from build123d import *

# Parameters (mm, degrees)
BOSS_EXTRUDE1_DEPTH     = 8
CUT_EXTRUDE1_DEPTH      = 2
CUT_EXTRUDE2_DEPTH      = 1
CUT_EXTRUDE2_DEPTH_BACK = 1
SKETCH7_R               = 0.5
BOSS_EXTRUDE4_DEPTH     = 30
CUT_EXTRUDE3_DEPTH      = 2


with BuildPart() as part:
    # Sketch1 → Boss-Extrude1 (new body)
    with BuildSketch(Plane(origin=(0, 0, 0), x_dir=(1, 0, 0), z_dir=(0, 1, 0))):
        with BuildLine():
            Line((12.297414328, 5.987472362), (16.301582158, 4.720916174))
            ThreePointArc((16.301582158, 4.720916174), (16.806716232, 4.358414998), (17, 3.767475981))
            Line((17, 3.767475981), (17, -3.767475981))
            ThreePointArc((17, -3.767475981), (16.806716232, -4.358414998), (16.301582158, -4.720916174))
            Line((16.301582158, -4.720916174), (12.297414328, -5.987472362))
            ThreePointArc((12.297414328, -5.987472362), (10.950566944, -6.649754843), (9.860946513, -7.68190952))
            ThreePointArc((9.860946513, -7.68190952), (-12.5, 0), (9.860946513, 7.68190952))
            ThreePointArc((9.860946513, 7.68190952), (10.950566944, 6.649754843), (12.297414328, 5.987472362))
        make_face()
    extrude(amount=BOSS_EXTRUDE1_DEPTH)

    # Sketch2 → Cut-Extrude1 (cut)
    with BuildSketch(Plane.XZ):
        with BuildLine():
            Line((1, 11.25), (1, 12.459935794))
            ThreePointArc((1, 12.459935794), (0, 12.5), (-1, 12.459935794))
            Line((-1, 12.459935794), (-1, 11.25))
            ThreePointArc((-1, 11.25), (0, 10.25), (1, 11.25))
        make_face()
        with BuildLine():
            Line((-11.25, -1), (-12.459935794, -1))
            ThreePointArc((-12.459935794, -1), (-12.5, 0), (-12.459935794, 1))
            Line((-12.459935794, 1), (-11.25, 1))
            ThreePointArc((-11.25, 1), (-10.25, 0), (-11.25, -1))
        make_face()
        with BuildLine():
            Line((1, -11.25), (1, -12.459935794))
            ThreePointArc((1, -12.459935794), (0, -12.5), (-1, -12.459935794))
            Line((-1, -12.459935794), (-1, -11.25))
            ThreePointArc((-1, -11.25), (0, -10.25), (1, -11.25))
        make_face()
    extrude(amount=-CUT_EXTRUDE1_DEPTH, mode=Mode.SUBTRACT)

    # Sketch3 → Cut-Extrude2 (cut, two sides: drawn at the far end of the back side and taken through both)
    with BuildSketch(Plane.XY.offset(-CUT_EXTRUDE2_DEPTH_BACK)):
        with BuildLine():
            Line((16, 0), (14.339588828, 3.617029189))
            ThreePointArc((14.339588828, 3.617029189), (14.248707164, 3.675309612), (14.1578255, 3.617029189))
            Line((14.1578255, 3.617029189), (12.497414328, 0))
            Line((12.497414328, 0), (16, 0))
        make_face()
    extrude(amount=CUT_EXTRUDE2_DEPTH + CUT_EXTRUDE2_DEPTH_BACK, mode=Mode.SUBTRACT)

    # Sketch6 → Cut-Revolve3 (revolve, cut)
    with BuildSketch(Plane.XY, mode=Mode.PRIVATE) as cut_revolve3_sk:
        with BuildLine():
            Line((-9.049917084, 8), (-0.023760171, 8))
            ThreePointArc((-0.023760171, 8), (-0.315220074, 7.915431347), (-0.516149554, 7.687993274))
            Line((-0.516149554, 7.687993274), (-2.834306132, 7.687993274))
            ThreePointArc((-2.834306132, 7.687993274), (-3.046438167, 7.600125308), (-3.134306132, 7.387993274))
            Line((-3.134306132, 7.387993274), (-3.134306132, 5.033771489))
            ThreePointArc((-3.134306132, 5.033771489), (-3.222174098, 4.821639455), (-3.434306132, 4.733771489))
            Line((-3.434306132, 4.733771489), (-5.381583428, 4.733771489))
            ThreePointArc((-5.381583428, 4.733771489), (-5.593715462, 4.821639455), (-5.681583428, 5.033771489))
            Line((-5.681583428, 5.033771489), (-5.681583428, 7.387993274))
            ThreePointArc((-5.681583428, 7.387993274), (-5.769451393, 7.600125308), (-5.981583428, 7.687993274))
            Line((-5.981583428, 7.687993274), (-9.049917084, 7.687993274))
            Line((-9.049917084, 7.687993274), (-9.049917084, 8))
        make_face()
    revolve(cut_revolve3_sk.sketch.rotate(Axis((0, 0, 0), (0, 1, 0)), 270), axis=Axis((0, 0, 0), (0, 1, 0)), mode=Mode.SUBTRACT)

    # Sketch7 → Boss-Extrude4 (add)
    with BuildSketch(Plane(origin=(17, 0, 0), x_dir=(0, 0, -1), z_dir=(1, 0, 0))):
        with Locations(Location((-1.563421987, 4, 0), (0, 0, 180))):
            Circle(SKETCH7_R)
        with Locations(Location((-0.553421987, 4, 0), (0, 0, 180))):
            Circle(SKETCH7_R)
        with Locations(Location((0.456578013, 4, 0), (0, 0, 180))):
            Circle(SKETCH7_R)
        with Locations(Location((1.466578013, 4, 0), (0, 0, 180))):
            Circle(SKETCH7_R)
    extrude(amount=BOSS_EXTRUDE4_DEPTH)

    # Sketch8 → Cut-Extrude3 (cut)
    with BuildSketch(Plane(origin=(0, 8, 0), x_dir=(1, 0, 0), z_dir=(0, 1, 0))):
        with BuildLine():
            ThreePointArc((-11.496633178, -3.033982251), (-11.890232168, -0.001304237), (-11.497298495, 3.031460051))
            ThreePointArc((-11.497298495, 3.031460051), (-10.953844404, 3.348128163), (-10.637176292, 2.804674072))
            ThreePointArc((-10.637176292, 2.804674072), (-11.000714274, 0.001254503), (-10.637815696, -2.802247907))
            ThreePointArc((-10.637815696, -2.802247907), (-10.951370221, -3.347475805), (-11.496633178, -3.033982251))
        make_face()
        with BuildLine():
            ThreePointArc((3.120810885, 11.473367515), (5.943986582, 10.297895233), (8.373970662, 8.441222546))
            ThreePointArc((8.373970662, 8.441222546), (8.376486246, 7.812243441), (7.747507142, 7.809727858))
            ThreePointArc((7.747507142, 7.809727858), (5.501443569, 9.52627077), (2.892089973, 10.613742587))
            ThreePointArc((2.892089973, 10.613742587), (2.576686025, 11.15790272), (3.120810885, 11.473367515))
        make_face()
        with BuildLine():
            ThreePointArc((8.375822292, -8.439385265), (5.946245587, -10.296590996), (3.123327833, -11.472682597))
            ThreePointArc((3.123327833, -11.472682597), (2.577358158, -11.160371604), (2.889669151, -10.614401929))
            ThreePointArc((2.889669151, -10.614401929), (5.499270705, -9.527525273), (7.745725723, -7.81149468))
            ThreePointArc((7.745725723, -7.81149468), (8.374684196, -7.810426915), (8.375822292, -8.439385265))
        make_face()
    extrude(amount=-CUT_EXTRUDE3_DEPTH, mode=Mode.SUBTRACT)


solid = part.part
Geometry check sheet. Reference: the model listing, model coordinates, mm. A direction names the side the tool comes from. Coordinates: 2 decimals unless noted, no trailing zeros. Order: outer loops, then holes, each group sorted by start corner. A loop starts at its lowest first (then second) coordinate and runs counter-clockwise, first axis right, second up. Notation, with made-up numbers: (73.5, 78) - (123.5, 78) arc R23 ccw to (123.5, 94) - close; hole circle Ø6 at (13, 45). An arc over 180 degrees is marked (long way). Answer in a Markdown table with one row per item. Add a question column.
1) Material ranges on line 1 along Z through (x, y) = (5, 7); line 2 along Z through (x, y) = (0.5, 2.5); line 3 along Z through (x, y) = (6.5, 7.25) (3 decimals), recorded low to high. Write a range as [from, to].
2) Release check for a two-part mould opening along Z. For faces 1 (the flat face through (14.328, 3.944, 5.345)), 2 (the flat face through (9, 8, 3)), 3 (the flat face through (-12, 1, 1)), 4 (the cylindrical face through (10.933, 3.944, -6.662)) record: +Z half, -Z half, draft (parallel to the pull), parting line (faces both ways), or undercut.
3) Cross-section at A-A, the plane x = 11.5. Record the cut outline in (y, z), then the cut area to 3 significant figures.
4) Gauge pin test, flat ends, axial feed: P1, Ø1.3, axis at y = 0.5, z = 12, coming from the -X side; P2, Ø8, axis at x = 31.5, z = -3.5, coming from the +Y side; P3, Ø1.8, axis at x = 13.5, y = 2.5, coming from the -Z side. Record the tip position at first contact, or that the pin passes through.
5) Set-up check for faces 5 (the flat face through (0, 2, 11)), 6 (the cylindrical face through (5.536, 7.014, -9.506)), 7 (the flat face through (-1, 1, -12)): record each of +Z, -Z, +X, -X, +Y, -Y from which the full face is reachable in a straight line by a thin tool's end or side.
Check result:
| question | item | result |
|---|---|---|
| 1 | line 1 | z = [-11.46, -10.79], [-9.8, -2.7], [2.7, 9.8], [10.79, 11.46] |
| 1 | line 2 | z = [-12.49, 12.49] |
| 1 | line 3 | z = [-10.677, -9.956], [-8.875, 8.875], [9.956, 10.677] |
| 2 | face 1 | +Z half |
| 2 | face 2 | draft |
| 2 | face 3 | undercut |
| 2 | face 4 | -Z half |
| 3 | outline | (0, -6.32) - (8, -6.32) - (8, 6.32) - (0, 6.32) - close |
| 3 | area | 101 mm² |
| 4 | P1 | stops at x = -5.24 |
| 4 | P2 | stops at y = 4.5 |
| 4 | P3 | stops at z = -5.89 |
| 5 | face 5 | +Z, -Y |
| 5 | face 6 | +Y |
| 5 | face 7 | -Z, -Y |
